from build123d import *

# Parameters (mm, degrees)
SKETCH1_R           = 1.65
BOSS_EXTRUDE1_DEPTH = 3.175
SKETCH2_W           = 1
SKETCH2_H           = 172.53
BOSS_EXTRUDE2_DEPTH = 5.08
SKETCH4_R           = 1.75
BOSS_EXTRUDE3_DEPTH = 3.5
BOSS_EXTRUDE4_START = 1.6764
SKETCH5_R           = 3.048
SKETCH5_R_2         = 1.75
SKETCH5_R_3         = 3.998686497
BOSS_EXTRUDE4_DEPTH = 1.6764
SKETCH6_R           = 1.75
BOSS_EXTRUDE5_DEPTH = 4
SKETCH7_R           = 1.75
CUT_EXTRUDE1_DEPTH  = 4.54
SKETCH8_R           = 1.75
CUT_EXTRUDE2_DEPTH  = 162.599778233


with BuildPart() as part:
    # Sketch1 → Boss-Extrude1 (new body)
    with BuildSketch(Plane.XY):
        with BuildLine():
            Line((13.6, 160.665), (-11.6, 160.665))
            ThreePointArc((-11.6, 160.665), (-12.943502884, 160.108502884), (-13.5, 158.765))
            Line((-13.5, 158.765), (-13.5, -9.965))
            ThreePointArc((-13.5, -9.965), (-12.943502884, -11.308502884), (-11.6, -11.865))
            Line((-11.6, -11.865), (13.6, -11.865))
            ThreePointArc((13.6, -11.865), (14.943502884, -11.308502884), (15.5, -9.965))
            Line((15.5, -9.965), (15.5, 158.765))
            ThreePointArc((15.5, 158.765), (14.943502884, 160.108502884), (13.6, 160.665))
        make_face()
        with Locations(Location((-9.85, -4.975, 0), (0, 0, 180))):
            Circle(SKETCH1_R, mode=Mode.SUBTRACT)
        with Locations(Location((-9.85, 26.775, 0), (0, 0, 180))):
            Circle(SKETCH1_R, mode=Mode.SUBTRACT)
        with Locations(Location((11.85, -4.975, 0), (0, 0, 180))):
            Circle(SKETCH1_R, mode=Mode.SUBTRACT)
        with Locations(Location((11.85, 26.775, 0), (0, 0, 180))):
            Circle(SKETCH1_R, mode=Mode.SUBTRACT)
        with Locations(Location((-9.85, 122.025, 0), (0, 0, 180))):
            Circle(SKETCH1_R, mode=Mode.SUBTRACT)
        with Locations(Location((-9.85, 153.775, 0), (0, 0, 180))):
            Circle(SKETCH1_R, mode=Mode.SUBTRACT)
        with Locations(Location((11.85, 122.025, 0), (0, 0, 180))):
            Circle(SKETCH1_R, mode=Mode.SUBTRACT)
        with Locations(Location((11.85, 153.775, 0), (0, 0, 180))):
            Circle(SKETCH1_R, mode=Mode.SUBTRACT)
    extrude(amount=BOSS_EXTRUDE1_DEPTH)

    # Sketch2 → Boss-Extrude2 (add)
    with BuildSketch(Plane.XY.offset(3.175)):
        with Locations((1.5, 74.4)):
            Rectangle(SKETCH2_W, SKETCH2_H)
        with Locations((0.5, 74.4)):
            Rectangle(SKETCH2_W, SKETCH2_H)
    extrude(amount=BOSS_EXTRUDE2_DEPTH)

    # Sketch4 → Boss-Extrude3 (add)
    # profile 1 of 2: a face of its own
    with BuildSketch(Plane.ZY.offset(13.5)):
        with BuildLine():
            Line((8.82313313, 60.076784691), (3.175, 60.076784691))
            Line((3.175, 60.076784691), (3.175, 66.220321271))
            Line((3.175, 66.220321271), (8.765152639, 66.220321271))
            ThreePointArc((8.765152639, 66.220321271), (10.232903429, 63.162131486), (8.82313313, 60.076784691))
        make_face()
        with Locations((6.234395, 63.124395)):
            Circle(SKETCH4_R, mode=Mode.SUBTRACT)
    # profile 2 of 2: a face of its own
    with BuildSketch(Plane.ZY.offset(13.5)):
        with BuildLine():
            Line((8.799348167, 98.176497144), (3.175, 98.176497144))
            Line((3.175, 98.176497144), (3.175, 104.29693575))
            Line((3.175, 104.29693575), (8.769776515, 104.29693575))
            ThreePointArc((8.769776515, 104.29693575), (10.217897937, 101.243641784), (8.799348167, 98.176497144))
        make_face()
        with Locations((6.234395, 101.224395)):
            Circle(SKETCH4_R, mode=Mode.SUBTRACT)
    extrude(amount=-BOSS_EXTRUDE3_DEPTH)

    # Sketch5 → Boss-Extrude4 (add)
    # profile 1 of 2: a face of its own
    with BuildSketch(Plane.ZY.offset(13.5).offset(BOSS_EXTRUDE4_START)):
        with Locations(Location((6.234395, 101.224395, 0), (0, 0, 269.530929423))):
            Circle(SKETCH5_R)
        with Locations((6.234395, 101.224395)):
            Circle(SKETCH5_R_2, mode=Mode.SUBTRACT)
    # profile 2 of 2: a face of its own
    with BuildSketch(Plane.ZY.offset(13.5).offset(BOSS_EXTRUDE4_START)):
        with Locations((6.234395, 63.124395)):
            Circle(SKETCH5_R_3)
        with Locations((6.234395, 63.124395)):
            Circle(SKETCH5_R_2, mode=Mode.SUBTRACT)
    extrude(amount=-BOSS_EXTRUDE4_DEPTH)

    # Sketch6 → Boss-Extrude5 (add)
    # profile 1 of 2: a face of its own
    with BuildSketch(Plane.ZY.offset(-15.5)):
        with BuildLine():
            Line((7.145936701, 56.909889149), (3.175, 56.909889149))
            Line((3.175, 56.909889149), (3.175, 49.290110851))
            Line((3.175, 49.290110851), (7.204063299, 49.290110851))
            ThreePointArc((7.204063299, 49.290110851), (10.984889149, 53.129063299), (7.145936701, 56.909889149))
        make_face()
        with Locations((7.175, 53.1)):
            Circle(SKETCH6_R, mode=Mode.SUBTRACT)
    # profile 2 of 2: a face of its own
    with BuildSketch(Plane.ZY.offset(-15.5)):
        with BuildLine():
            Line((7.267081375, 97.90888711), (3.175, 97.90888711))
            Line((3.175, 97.90888711), (3.175, 90.29111289))
            Line((3.175, 90.29111289), (7.082918625, 90.29111289))
            ThreePointArc((7.082918625, 90.29111289), (10.98388711, 94.007918625), (7.267081375, 97.90888711))
        make_face()
        with Locations((7.175, 94.1)):
            Circle(SKETCH6_R, mode=Mode.SUBTRACT)
    extrude(amount=BOSS_EXTRUDE5_DEPTH)

    # Sketch7 → Cut-Extrude1 (cut)
    with BuildSketch(Plane.XY.offset(3.175)):
        with Locations((8.5, 74.4)):
            Circle(SKETCH7_R)
    extrude(amount=-CUT_EXTRUDE1_DEPTH, mode=Mode.SUBTRACT)

    # Sketch8 → Cut-Extrude2 (cut, through all)
    with BuildSketch(Plane.XY.offset(3.175)):
        with Locations((-6, 74.4)):
            Circle(SKETCH8_R)
    extrude(amount=-CUT_EXTRUDE2_DEPTH, mode=Mode.SUBTRACT)


solid = part.part
Geometry: final body of the model. Coordinates: model frame, mm. A direction names the side the tool comes from. Give positions to 0.01 mm unless a question says otherwise; leave off trailing zeros. Order: outer loops, then holes, each group sorted by start corner. A loop starts at its lowest first (then second) coordinate and runs counter-clockwise, first axis right, second up. Notation, with made-up numbers: (40, 6) -> (85, 6) arc R9 cw to (85, 14) -> close; hole circle Ø2 at (66.5, 70.25). An arc over 180 degrees is marked (long way). Put each result on its own line as item: value.
Q1. Section A-A, the plane y = 74.4. Return loops of the section in (x, z) (3 decimals), then the cut area to 3 significant figures.
Here are the results:
outline: (-13.5, 0) -> (-7.75, 0) -> (-7.75, 3.175) -> (-13.5, 3.175) -> close; (-4.25, 0) -> (6.75, 0) -> (6.75, 3.175) -> (2, 3.175) -> (2, 8.255) -> (0, 8.255) -> (0, 3.175) -> (-4.25, 3.175) -> close; (10.25, 0) -> (15.5, 0) -> (15.5, 3.175) -> (10.25, 3.175) -> close
area: 80.0 mm^2
Q2. Section B-B, the plane x = 8.5. Return loops of the section in (y, z) (3 decimals).
Here are the results:
outline: (-11.865, 0) -> (72.65, 0) -> (72.65, 3.175) -> (-11.865, 3.175) -> close; (76.15, 0) -> (160.665, 0) -> (160.665, 3.175) -> (76.15, 3.175) -> close
Q3. Draft query along Y for faces 1 (the face through (13.528, 53.045, 10.985)), 2 (the face through (2, 73, 6)), 3 (the face through (-12, 104.297, 6)). Return one class per face: released by +Y, released by -Y, zero draft, split by the parting line, or undercut.
Here are the results:
face 1: undercut
face 2: zero draft
face 3: released by +Y
Q4. Material intervals for L1, parallel to Y at x = -9.85, z = 2 (3 decimals); L2, parallel to X at y = 64.5, z = 3.5; L3, parallel to X at y = 56.5, z = 6.25, sorted ascending.
Here are the results:
L1: y = -11.865 to -6.625, -3.325 to 25.125, 28.425 to 120.375, 123.675 to 152.125, 155.425 to 160.665
L2: x = -15.18 to -10, 0 to 2
L3: x = 0 to 2, 11.5 to 15.5
Q5. Pin query (flat end, axial travel): pin 1 (1 mm diameter, centred on y = 42, z = 2, fed in from -X); pin 2 (1 mm diameter, centred on x = -12.5, z = 5.5, fed in from -Y); pin 3 (2 mm diameter, centred on x = 13, z = 4.5, fed in from +Y). Return the tip coordinate at first contact, or that it passes through.
Here are the results:
pin 1: stops at x = -13.5
pin 2: stops at y = 60.08
pin 3: stops at y = 97.91
Q6. Section C-C, the plane y = 94.1. Return loops of the section in (x, z) (3 decimals).
Here are the results:
outline: (-13.5, 0) -> (15.5, 0) -> (15.5, 5.425) -> (11.5, 5.425) -> (11.5, 3.175) -> (2, 3.175) -> (2, 8.255) -> (0, 8.255) -> (0, 3.175) -> (-13.5, 3.175) -> close; (11.5, 8.925) -> (15.5, 8.925) -> (15.5, 10.985) -> (11.5, 10.985) -> close
Q7. Reachability of faces 4 (the face through (-12.624, 99.516, 5.855)), 5 (the face through (14, 49.29, 5)), 6 (the face through (-12, 66.22, 6)) from +Z, -Z, +X, -X, +Y, -Y: full face, straight path, thin tool, end or side. Return the list, or none.
Here are the results:
face 4: -X
face 5: +Z, +X, -Y
face 6: +Z
Q8. Section D-D, the plane y = 17.5. Return loops of the section in (x, z) (3 decimals).
Here are the results:
outline: (-13.5, 0) -> (15.5, 0) -> (15.5, 3.175) -> (2, 3.175) -> (2, 8.255) -> (0, 8.255) -> (0, 3.175) -> (-13.5, 3.175) -> close
